Build history of the part. All positions in model axes, mm. A direction names the side the tool comes from. Round coordinates to 2 decimals unless told otherwise and drop trailing zeros. Loops run counter-clockwise (first coordinate to the right, second up) from the corner with the lowest first, then second, coordinate; pieces in that order, holes last. Notation, with made-up numbers: (74, 56.25) -> (98, 56.25) arc R12 ccw to (98, 78.25) -> close; hole circle Ø8 at (72.25, 44). An arc over 180 degrees is marked (long way). Put each result on its own line as item: value. Start each with the question number.
Item 1: Pull direction X, two halves, no side cores. Call faces 6 (the flat face through (1.5, -2, 17)), 7 (the flat face through (-4.5, -6, 2)), 8 (the flat face through (5.4, -0.1, 0)): +X half, -X half, draft (parallel to the pull), parting line (faces both ways), or undercut.
Item 2: Drill centre lines: probe 1 along Z at (x, y) = (-1, 1.5); probe 2 along Y at (x, z) = (6, 9.25); probe 3 along X at (y, z) = (-6.25, 2.75). Where is each one in solid material? Low to high. Write a range as [from, to].
Item 3: Flat gauge pins, fed straight in: pin 1 Ø1.6 at (x, z) = (-0.5, 7) entering from -Y; pin 2 Ø1.5 at (y, z) = (0.5, 5.5) entering from -X; pin 3 Ø8 at (y, z) = (-4.5, 9.5) entering from +X. Where does each tip first touch, or does it go through?
Item 4: Cut at B-B, the plane x = 0.5. List the corners of the cut face in (y, z), plus the area to 3 significant figures.
Item 5: Tool access for faces 1 (the flat face through (1.5, -2, 2)), 2 (the flat face through (-1, 6.8, 10)), 3 (the flat face through (-3, -6, 3)), 4 (the flat face through (-4, -5, 2)), 5 (the flat face through (2.5, 6, 10)): list every direction of +Z, -Z, +X, -X, +Y, -Y with a clear straight run to the whole face (end or side of a thin tool).
Item 6: Cut at A-A, the plane y = 6. List the corners of the cut face in (x, z), plus the area to 3 significant figures.
Item 7: Cut at C-C, the plane y = -1.5. Count the separate pieces of the cut face and the enclosed holes in it, plus the area to 3 significant figures.
```python
from build123d import *

# Parameters (mm, degrees)
AUFSATZ_LINEAR_AUSTRAGEN1_DEPTH = 20
SKIZZE2_W                       = 20
SKIZZE2_H                       = 3
AUFSATZ_LINEAR_AUSTRAGEN2_DEPTH = 3
SKIZZE3_W                       = 1.5
SKIZZE3_H                       = 20
SCHNITT_LINEAR_AUSTRAGEN1_DEPTH = 1.8
SKIZZE4_W                       = 1.5
SKIZZE4_H                       = 20
SCHNITT_LINEAR_AUSTRAGEN2_DEPTH = 1.8
SKIZZE14_W                      = 10
SKIZZE14_H                      = 13.6
SCHNITT_LINEAR_AUSTRAGEN5_DEPTH = 4
SKIZZE15_W                      = 10
SKIZZE15_H                      = 3
SCHNITT_LINEAR_AUSTRAGEN6_DEPTH = 6


# Read off the part's stored shape, not the designer's step: Aufsatz-Linear austragen1
with BuildPart() as part:
    # Aufsatz-Linear austragen1 outline → Aufsatz-Linear austragen1 (new body)
    with BuildSketch(Plane.XY):
        with BuildLine():
            Line((9.808332267, 5), (9.808332267, 4.212574368))
            add(Edge.make_bspline(
                [(9.808332267, 4.212574368), (1.184205361, -0.248328273), (6.5, -8)],
                knots=[0.083691521, 0.083691521, 0.083691521, 1, 1, 1], degree=2))
            Line((6.5, -8), (7.324710859, -7.434445405))
            add(Edge.make_bspline(
                [(11.5, 3.928207011), (11.209820184, 3.80014068), (10.506924616, 3.473790212), (9.167508184, 2.759616852), (7.676014914, 1.732695654), (6.437995439, 0.449518828), (5.702276721, -0.864348189), (5.405604765, -2.23902291), (5.529123845, -3.763138416), (6.029994776, -5.206555772), (6.676958994, -6.441666188), (7.105896283, -7.115968485), (7.324710859, -7.434445405)],
                knots=[0.019043297, 0.019043297, 0.019043297, 0.019043297, 0.0625, 0.125, 0.25, 0.375, 0.5, 0.625, 0.75, 0.875, 0.9375, 1, 1, 1, 1], degree=3))
            Line((11.5, 3.928207011), (11.5, 8))
            Line((11.5, 8), (-1.5, 8))
            Line((-1.5, 8), (-1.5, -8))
            Line((-1.5, -8), (1.5, -8))
            Line((1.5, -8), (1.5, 5))
            Line((1.5, 5), (9.808332267, 5))
        make_face()
    extrude(amount=AUFSATZ_LINEAR_AUSTRAGEN1_DEPTH)

    # Skizze2 → Aufsatz-Linear austragen2 (add)
    with BuildSketch(Plane.ZY.offset(1.5)):
        with Locations((10, 6.5)):
            Rectangle(SKIZZE2_W, SKIZZE2_H)
        with Locations((10, -6.5)):
            Rectangle(SKIZZE2_W, SKIZZE2_H)
    extrude(amount=AUFSATZ_LINEAR_AUSTRAGEN2_DEPTH)

    # Skizze3 → Schnitt-Linear austragen1 (cut)
    with BuildSketch(Plane.XZ.offset(-5)):
        with Locations((-2.25, 10)):
            Rectangle(SKIZZE3_W, SKIZZE3_H)
    extrude(amount=-SCHNITT_LINEAR_AUSTRAGEN1_DEPTH, mode=Mode.SUBTRACT)

    # Skizze4 → Schnitt-Linear austragen2 (cut)
    with BuildSketch(Plane(origin=(0, -5, 0), x_dir=(1, 0, 0), z_dir=(0, 1, 0))):
        with Locations((-2.25, -10)):
            Rectangle(SKIZZE4_W, SKIZZE4_H)
    extrude(amount=-SCHNITT_LINEAR_AUSTRAGEN2_DEPTH, mode=Mode.SUBTRACT)

    # Skizze14 → Schnitt-Linear austragen5 (cut)
    with BuildSketch(Plane.ZY.offset(1.5)):
        with Locations((10, 0)):
            Rectangle(SKIZZE14_W, SKIZZE14_H)
    extrude(amount=-SCHNITT_LINEAR_AUSTRAGEN5_DEPTH, mode=Mode.SUBTRACT)

    # Skizze15 → Schnitt-Linear austragen6 (cut)
    with BuildSketch(Plane.ZY.offset(4.5)):
        with Locations((10, -6.5)):
            Rectangle(SKIZZE15_W, SKIZZE15_H)
    extrude(amount=-SCHNITT_LINEAR_AUSTRAGEN6_DEPTH, mode=Mode.SUBTRACT)


solid = part.part
```
Reply:
1. face 6: undercut
1. face 7: -X half
1. face 8: draft
2. probe 1: z = [0, 5], [15, 20]
2. probe 2: y = [-7.23, -5.04], [-0.38, 1.37], [5, 8]
2. probe 3: x = [-4.5, -3], [-1.5, 1.5], [5.46, 6.59]
3. pin 1: stops at y = 6.8
3. pin 2: stops at x = -1.5
3. pin 3: stops at x = 7.32
4. outline: (-8, 0) -> (8, 0) -> (8, 20) -> (-8, 20) -> (-8, 15) -> (6.8, 15) -> (6.8, 5) -> (-8, 5) -> close
4. area: 172 mm^2
5. face 1: +Z, -Z, -Y
5. face 2: none
5. face 3: +Z, -Z
5. face 4: +Z, -Z, -X
5. face 5: -Y
6. outline: (-4.5, 0) -> (-3, 0) -> (-3, 20) -> (-4.5, 20) -> close; (-1.5, 0) -> (11.5, 0) -> (11.5, 20) -> (-1.5, 20) -> (-1.5, 15) -> (2.5, 15) -> (2.5, 5) -> (-1.5, 5) -> close
6. area: 250 mm^2
7. separate pieces: 3
7. enclosed holes: 0
7. area: 50.3 mm^2
